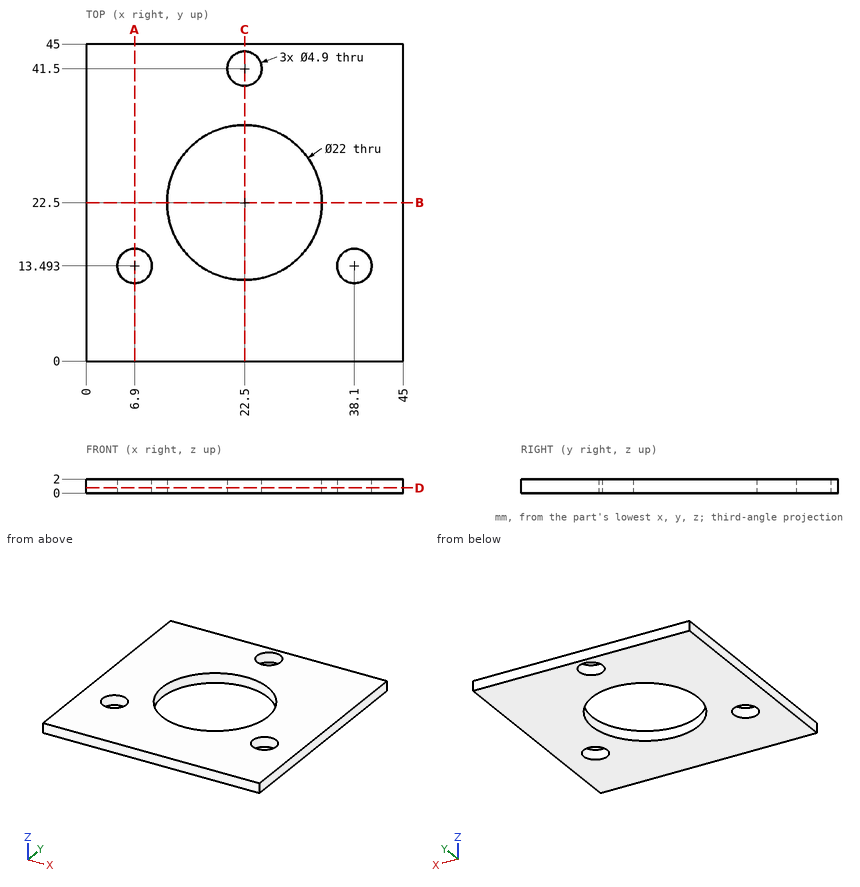
Print and shaded views of the part. All mm, measured from the part's lowest x, y and z. Coordinates: 2 decimals unless noted, no trailing zeros. Order: outer loops, then holes, each group sorted by start corner. A loop starts at its lowest first (then second) coordinate and runs counter-clockwise, first axis right, second up.
(1) Slice it at A-A, the plane x = 6.9. Write the cut outline in (y, z).
Check sheet entries:
outline: (0, 0) - (11.04, 0) - (11.04, 2) - (0, 2) - close; (15.94, 0) - (45, 0) - (45, 2) - (15.94, 2) - close
(2) Probe L1, parallel to Y at x = 22.5, z = 1.45; L2, parallel to X at y = 22.5, z = 1.45; L3, parallel to Y at x = 6.9, z = 0.6. List the from-to ranges inside material, lowest first.
Check sheet entries:
L1: y = 0 to 11.5, 33.5 to 39.05, 43.95 to 45
L2: x = 0 to 11.5, 33.5 to 45
L3: y = 0 to 11.04, 15.94 to 45
(3) Slice it at C-C, the plane x = 22.5. Write the cut outline in (y, z).
Check sheet entries:
outline: (0, 0) - (11.5, 0) - (11.5, 2) - (0, 2) - close; (33.5, 0) - (39.05, 0) - (39.05, 2) - (33.5, 2) - close; (43.95, 0) - (45, 0) - (45, 2) - (43.95, 2) - close
(4) Slice it at B-B, the plane y = 22.5. Write the cut outline in (x, z).
Check sheet entries:
outline: (0, 0) - (11.5, 0) - (11.5, 2) - (0, 2) - close; (33.5, 0) - (45, 0) - (45, 2) - (33.5, 2) - close
(5) Pin check, flat tip, straight feed: pin 1 Ø10 at (x, y) = (36.5, 9.5) entering from -Z. Stop position of the tip, or through.
Check sheet entries:
pin 1: stops at z = 0
(6) Slice it at D-D, the plane z = 0.75. Write the cut outline in (x, y).
Check sheet entries:
outline: (0, 0) - (45, 0) - (45, 45) - (0, 45) - close; hole circle Ø4.9 at (6.9, 13.49); hole circle Ø22 at (22.5, 22.5); hole circle Ø4.9 at (22.5, 41.5); hole circle Ø4.9 at (38.1, 13.49)
